from build123d import *

# Parameters (mm, degrees)
F0_W     = 125.8938722312
F0_H     = 62.8035478294
F0_W_2   = 4.9569368675
F0_H_2   = 42.6520612952
F1_DEPTH = 20


with BuildPart() as f1:
    # F0 (on Front) → F1 (new body)
    with BuildSketch(Plane.XZ):
        with Locations((2.0074192435, 2.8677415103)):
            Rectangle(F0_W, F0_H)
        Polygon((-28.719614941, -15.4966360104), (-28.719614941, -19.9308074079), (-52.4961087293, -19.9308074079), (-52.4961087293, 22.7212538872), (-28.719614941, 22.7212538872), (-28.719614941, 18.3150877828), (-47.5391718618, 18.3150877828), (-47.5391718618, 4.5738239993), (-29.8584968578, 4.5738239993), (-29.8584968578, 0.1956631879), (-47.5391718618, 0.1956631879), (-47.5391718618, -15.4966360104), align=None, mode=Mode.SUBTRACT)
        with BuildLine():
            Line((-4.6537331246, -4.7052630936), (5.0921088522, 22.7212538872))
            Line((5.0921088522, 22.7212538872), (10.4224496269, 22.7212538872))
            Line((10.4224496269, 22.7212538872), (-4.9431211527, -19.9308074079))
            Line((-4.9431211527, -19.9308074079), (-9.8440474341, -19.9308074079))
            Line((-9.8440474341, -19.9308074079), (-25.1349374323, 22.7212538872))
            Line((-25.1349374323, 22.7212538872), (-19.879277439, 22.7212538872))
            Line((-19.879277439, 22.7212538872), (-10.0774248761, -4.8732948518))
            add(Edge.make_bspline(
                [(-10.0774248761, -4.8732948518), (-8.3877721962, -9.634194668), (-7.3982518423, -14.1243766516)],
                knots=[0, 0, 0, 1, 1, 1], degree=2))
            add(Edge.make_bspline(
                [(-7.3982518423, -14.1243766516), (-6.3433858045, -9.4008172261), (-4.6537331246, -4.7052630936)],
                knots=[0, 0, 0, 1, 1, 1], degree=2))
        make_face(mode=Mode.SUBTRACT)
        with Locations((18.763359403, 1.3952232396)):
            Rectangle(F0_W_2, F0_H_2, mode=Mode.SUBTRACT)
        Polygon((56.7151990169, -15.4966360104), (56.7151990169, -19.9308074079), (32.9387052285, -19.9308074079), (32.9387052285, 22.7212538872), (56.7151990169, 22.7212538872), (56.7151990169, 18.3150877828), (37.8956420961, 18.3150877828), (37.8956420961, 4.5738239993), (55.5763171, 4.5738239993), (55.5763171, 0.1956631879), (37.8956420961, 0.1956631879), (37.8956420961, -15.4966360104), align=None, mode=Mode.SUBTRACT)
    extrude(amount=F1_DEPTH)


solid = f1.part
Can you work these out from the model? Positions are in its coordinate system, mm. Round coordinates to 2 decimals unless told otherwise and drop trailing zeros. Loops run counter-clockwise (first coordinate to the right, second up) from the corner with the lowest first, then second, coordinate; pieces in that order, holes last. Notation, with made-up numbers: (-3.75, -13) - (40.25, -13) arc R22 cw to (40.25, 25) - close; hole circle Ø5 at (41.25, 82.25). An arc over 180 degrees is marked (long way). Use CSV: the item, a comma, the result in double quotes. Start each with the question number.
1) If we section it at C-C on z = 1.5: Write out the boundary of the cut face in (x, y).
2) If we section it at A-A on x = -35.5: Write out the boundary of the cut face in (y, z), plus the area to 3 significant figures.
3) If we section it at B-B on x = 19: Write out the boundary of the cut face in (y, z).
4) We'd pull the mould along X, two halves only. Please class faces 1 (the flat face through (16.285, -10, 1)), 2 (the flat face through (1, -10, -28.534)): released by +X, released by -X, zero draft, split by the parting line, or undercut.
5) If we section it at D-D on y = -14.25: Count the separate pieces of the cut face and the enclosed holes in it, plus the area to 3 significant figures.
6) Please list where these lines run through material, in increasing order: probe 1 along Z at (x, y) = (-42.5, -9.5); probe 2 along X at (y, z) = (-13.5, -6); probe 3 along X at (y, z) = (-7.5, 20). Write a range as [from, to].
Geometry results:
1,outline,"(-60.94, -20) - (-52.5, -20) - (-52.5, 0) - (-60.94, 0) - close; (-29.86, -20) - (-17.53, -20) - (-17.53, 0) - (-29.86, 0) - close; (-12.34, -20) - (-2.45, -20) - (-2.45, 0) - (-12.34, 0) - close; (2.78, -20) - (16.28, -20) - (16.28, 0) - (2.78, 0) - close; (21.24, -20) - (32.94, -20) - (32.94, 0) - (21.24, 0) - close; (55.58, -20) - (64.95, -20) - (64.95, 0) - (55.58, 0) - close"
2,outline,"(-20, -28.53) - (0, -28.53) - (0, -19.93) - (-20, -19.93) - close; (-20, -15.5) - (0, -15.5) - (0, 0.2) - (-20, 0.2) - close; (-20, 4.57) - (0, 4.57) - (0, 18.32) - (-20, 18.32) - close; (-20, 22.72) - (0, 22.72) - (0, 34.27) - (-20, 34.27) - close"
2,area,"992 mm2"
3,outline,"(-20, -28.53) - (0, -28.53) - (0, -19.93) - (-20, -19.93) - close; (-20, 22.72) - (0, 22.72) - (0, 34.27) - (-20, 34.27) - close"
4,face 1,"undercut"
4,face 2,"zero draft"
5,separate pieces,"1"
5,enclosed holes,"4"
5,area,"6,360 mm2"
6,probe 1,"z = [-28.53, -19.93], [-15.5, 0.2], [4.57, 18.32], [22.72, 34.27]"
6,probe 2,"x = [-60.94, -52.5], [-47.54, -14.84], [-9.69, -5.11], [0.08, 16.28], [21.24, 32.94], [37.9, 64.95]"
6,probe 3,"x = [-60.94, -52.5], [-28.72, -24.16], [-18.91, 4.13], [9.44, 16.28], [21.24, 32.94], [56.72, 64.95]"
